Design review of the part built by this model. Coordinates are the model's own, in mm. Face numbers are marked on the shaded views. A direction names the side the tool comes from. Coordinates: 2 decimals unless noted, no trailing zeros. Order: outer loops, then holes, each group sorted by start corner. A loop starts at its lowest first (then second) coordinate and runs counter-clockwise, first axis right, second up. Notation, with made-up numbers: M 79.5,65 L 95.5,65 A21 cw 95.5,76 Z; hole C 82.5,51 d5. An arc over 180 degrees is marked long. Answer in a Markdown table with one row per item.
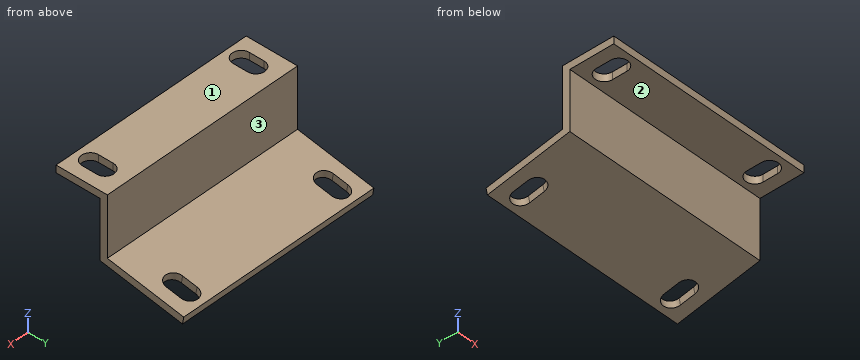
from build123d import *

# Parameters (mm, degrees)
EXTRUDE_1_DEPTH     = 70
CUT_EXTRUDE_1_DEPTH = 70
CUT_EXTRUDE_2_DEPTH = 10


with BuildPart() as part:
    # 草图1 → 凸台-拉伸1 (new body)
    with BuildSketch(Plane(origin=(0, 0, 0), x_dir=(0, 0, -1), z_dir=(1, 0, 0))):
        Polygon((0, 0), (20, 0), (24.957460038, 28.115152986), (22.495440656, 28.54927343), (17.902250922, 2.5), (-2.5, 2.5), (-2.5, -15), (0, -15), align=None)
    extrude(amount=EXTRUDE_1_DEPTH)

    # 草图2 → 切除-拉伸1 (cut)
    with BuildSketch(Plane.XY.offset(2.5)):
        with BuildLine():
            Line((4.25, -10), (4.25, -5))
            ThreePointArc((4.25, -5), (7.25, -2), (10.25, -5))
            Line((10.25, -5), (10.25, -10))
            ThreePointArc((10.25, -10), (7.25, -13), (4.25, -10))
        make_face()
        with BuildLine():
            Line((65.75, -10), (65.75, -5))
            ThreePointArc((65.75, -5), (62.75, -2), (59.75, -5))
            Line((59.75, -5), (59.75, -10))
            ThreePointArc((59.75, -10), (62.75, -13), (65.75, -10))
        make_face()
    extrude(amount=-CUT_EXTRUDE_1_DEPTH, mode=Mode.SUBTRACT)

    # 草图3 → 切除-拉伸2 (cut)
    with BuildSketch(Plane(origin=(0, -2.986080989, -16.934906825), x_dir=(1, 0, 0), z_dir=(0, 0.17364817766693397, 0.9848077530122076))):
        with BuildLine():
            Line((4.25, 26.994852841), (4.25, 21.994852841))
            ThreePointArc((4.25, 21.994852841), (7.25, 18.994852841), (10.25, 21.994852841))
            Line((10.25, 21.994852841), (10.25, 26.994852841))
            ThreePointArc((10.25, 26.994852841), (7.25, 29.994852841), (4.25, 26.994852841))
        make_face()
        with BuildLine():
            Line((59.75, 26.994852841), (59.75, 21.994852841))
            ThreePointArc((59.75, 21.994852841), (62.75, 18.994852841), (65.75, 21.994852841))
            Line((65.75, 21.994852841), (65.75, 26.994852841))
            ThreePointArc((65.75, 26.994852841), (62.75, 29.994852841), (59.75, 26.994852841))
        make_face()
    extrude(amount=-CUT_EXTRUDE_2_DEPTH, mode=Mode.SUBTRACT)


solid = part.part
(1) For line 1 along Y through (x, z) = (39.5, -4); line 2 along Y through (x, z) = (42, 1.75); line 3 along X through (y, z) = (-12.5, 1.5), list the stretches that pass through material, from the lowest coordinate up. Write a range as from..to.
Return value:
| item | result |
|---|---|
| line 1 | y = 0..2.5 |
| line 2 | y = -15..2.5 |
| line 3 | x = 0..5.59, 8.91..61.09, 64.41..70 |
(2) Add section A-A, the plane y = -9. Give the boundary of the cut face in (x, z).
Return value:
| item | result |
|---|---|
| outline | M 0,0 L 4.25,0 L 4.25,2.5 L 0,2.5 Z; M 10.25,0 L 59.75,0 L 59.75,2.5 L 10.25,2.5 Z; M 65.75,0 L 70,0 L 70,2.5 L 65.75,2.5 Z |
(3) Add section B-B, the plane x = 9. Give the boundary of the cut face in (y, z).
Return value:
| item | result |
|---|---|
| outline | M -15,0 L -12.44,0 L -12.44,2.5 L -15,2.5 Z; M -2.56,0 L 0,0 L 0,-20 L 15.84,-22.79 L 16.27,-20.33 L 2.5,-17.9 L 2.5,2.5 L -2.56,2.5 Z; M 25.56,-24.51 L 28.12,-24.96 L 28.55,-22.5 L 26,-22.05 Z |
(4) Insertion check: pin 1 Ø4 at (x, y) = (12.5, 13) entering from -Z; pin 2 Ø7.5 at (x, y) = (51, -9.5) entering from -Z; pin 3 Ø6 at (x, y) = (31.5, 14.5) entering from +Z. Each pin has a flat end and moves straight along its axis. Give the tip position at first contact, or say it passes through.
Return value:
| item | result |
|---|---|
| pin 1 | stops at z = -22.64 |
| pin 2 | stops at z = 0 |
| pin 3 | stops at z = -19.49 |
(5) Add section D-D, the plane z = -7.5. Give the boundary of the cut face in (x, y), and give its area (3 significant figures).
Return value:
| item | result |
|---|---|
| outline | M 0,0 L 70,0 L 70,2.5 L 0,2.5 Z |
| area | 175 mm2 |
(6) Add section C-C, the plane x = 59. Give the boundary of the cut face in (y, z), and give its area (3 significant figures).
Return value:
| item | result |
|---|---|
| outline | M -15,0 L 0,0 L 0,-20 L 28.12,-24.96 L 28.55,-22.5 L 2.5,-17.9 L 2.5,2.5 L -15,2.5 Z |
| area | 160 mm2 |
(7) For the marked faces 1, 2 and 3, list the 3-axis set-ups (+Z, -Z, +X, -X, +Y, -Y) from which the entire face can be reached by the end or side of a thin tool; tool diameter is ignored.
Return value:
| item | result |
|---|---|
| face 1 | +Z, +X, -X, +Y, -Y |
| face 2 | -Z, +X, -X, -Y |
| face 3 | +Z, +X, -X, +Y |
